Autodesk Inventor part; units mm, degrees
ref_plane "YZ Plane" through (0, 0, 0) normal (1, 0, 0) x (0, 1, 0)
ref_plane "XZ Plane" through (0, 0, 0) normal (0, 1, 0) x (-1, 0, 0)
ref_plane "XY Plane" through (0, 0, 0) normal (0, 0, 1) x (1, 0, 0)
sketch "skt_base" plane through (0, 0, 0) normal (0, 0, 1) x (1, 0, 0)
  line L0 (-30, -8.25) -> (30, -8.25)
  line L1 (30, -8.25) -> (30, 8.25)
  line L2 (30, 8.25) -> (-30, 8.25)
  line L3 (-30, 8.25) -> (-30, -8.25)
  line L4 (-30, -8.25) -> (30, 8.25) construction
  line L5 (30, -8.25) -> (-30, 8.25) construction
  line L6 (-30, 0) -> (30, 0) construction
  line L7 (0, -8.25) -> (0, 8.25) construction
  line L8 (14.5, 0) -> (23.5, 0) construction
  line L9 (16.75, -2.25) -> (21.25, -2.25)
  line L10 (21.25, 2.25) -> (16.75, 2.25)
  arc A0 (16.75, 2.25) -> (16.75, -2.25) centre (16.75, 0) ccw
  arc A1 (21.25, -2.25) -> (21.25, 2.25) centre (21.25, 0) ccw
  line L11 (12.5, 0) -> (25.5, 0) construction
  line L12 (16.75, -4.25) -> (21.25, -4.25)
  line L13 (21.25, 4.25) -> (16.75, 4.25)
  arc A2 (16.75, 4.25) -> (16.75, -4.25) centre (16.75, 0) ccw
  arc A3 (21.25, -4.25) -> (21.25, 4.25) centre (21.25, 0) ccw
  line L14 (-16.75, -2.25) -> (-21.25, -2.25)
  line L15 (-21.25, 2.25) -> (-16.75, 2.25)
  arc A4 (-16.75, -2.25) -> (-16.75, 2.25) centre (-16.75, 0) ccw
  arc A5 (-21.25, 2.25) -> (-21.25, -2.25) centre (-21.25, 0) ccw
  line L16 (-16.75, -4.25) -> (-21.25, -4.25)
  line L17 (-21.25, 4.25) -> (-16.75, 4.25)
  arc A6 (-16.75, -4.25) -> (-16.75, 4.25) centre (-16.75, 0) ccw
  arc A7 (-21.25, 4.25) -> (-21.25, -4.25) centre (-21.25, 0) ccw
  circle A8 centre (0, 0) radius 3.75
  circle A9 centre (0, 0) radius 6
  circle A10 centre (0, 0) radius 8
  point P0 (0, 0)
  point P1 (19, 0)
  point P2 (19, 0)
  point P3 (0, 0)
  dimension "d13" = 60
  dimension "d14" = 16.5
  dimension "d29" = 6.5
  dimension "d30" = 4.5
  dimension "d31" = 9
  dimension "d32" = 2
  dimension "d33" = 2
  dimension "d47" = 16
  dimension "d48" = 12
  dimension "d49" = 7.5
extrude "base" add sketch "skt_base" along normal blind 3.5 contours L3 L2 L1 L0
extrude "screw_head" add sketch "skt_base" along normal blind 1.75 contours A2 L13 A3 L12 | L16 A7 L17 A6
extrude "handle_support" add sketch "skt_base" along normal blind 7 contours A10
extrude "handle_guide" add sketch "skt_base" along normal blind 5.5 contours A9
extrude "handle_screw_head" cut sketch "skt_base" along normal blind 3.7 contours A9
fillet "side_fillets" radius 4 4 edges at (-30, -8.25, 1.75) (30, -8.25, 1.75) (30, 8.25, 1.75) (-30, 8.25, 1.75)
equation "\"d13\" = base_l"
equation "\"d14\" = base_w"
equation "\"d29\" = base_screw_b"
equation "\"d30\" = base_screw_w"
equation "\"d31\" = base_screw_l"
equation "\"d32\" = base_screw_p"
equation "\"d33\" = base_screw_p"
equation "\"d47\" = handle_screw_e"
equation "\"d48\" = handle_screw_p"
equation "\"d49\" = handle_screw_d"
equation "\"d15\" = base_t"
equation "\"d34\" = base_screw_t"
equation "\"d50\" = handle_screw_h"
equation "\"d52\" = handle_screw_h - handle_screw_b"
equation "\"d54\" = handle_screw_h - 2.2 * handle_screw_b"
equation "\"wall_inner_diam\" = 2"
equation "\"wall_outer_diam\" = 1"
equation "\"wall_height\" = 8"
equation "\"leg_diam\" = 3"
equation "\"leg_height\" = 4"
equation "\"wall_widh\" = 8"
equation "\"base_screw_w\" = 4.5"
equation "\"base_t\" = 3.5"
equation "\"base_w\" = 16.5"
equation "\"base_l\" = 60"
equation "\"base_screw_p\" = 2"
equation "\"base_screw_l\" = 9"
equation "\"base_screw_t\" = 1.75"
equation "\"base_screw_b\" = 6.5"
equation "\"handle_screw_p\" = 12"
equation "\"handle_screw_d\" = 7.5"
equation "\"handle_screw_e\" = 16"
equation "\"handle_screw_b\" = 1.5"
equation "\"handle_screw_h\" = 7"
equation "\"d44\" = 7.5"
equation "\"d45\" = 16"
equation "\"d46\" = 12"
properties part number "coffee"
Could you check a few things on this model? Use its own coordinates, in mm. A direction names the side the tool comes from. Coordinates: 2 decimals unless noted, no trailing zeros. Write each loop counter-clockwise with the first axis right and the second up, starting at its lowest first coordinate (ties: lowest second). Pieces come first, ordered by that corner, then holes. Notation, with made-up numbers: (18.25, 74.5) - (57.25, 74.5) arc R22 ccw to (57.25, 93.5) - close; hole circle Ø9 at (-22, 23.25). An arc over 180 degrees is marked (long way). Put each result on its own line as item: value. Start each with the question number.
Q1. I want a section at C-C on x = -11.5. Write out the boundary of the cut face in (y, z).
Q2. I want a section at B-B on x = 2.5. Write out the boundary of the cut face in (y, z).
Q3. Thinking about a two-plate mould opening in Y: for faces 1 (the cylindrical face through (23.5, 0, 0.9)), 2 (the cylindrical face through (28.859, 7.047, 1.774)), 3 (the flat face through (-2, 6, 7)), which applies, pulls with the +Y half, pulls with the -Y half, needs draft (parallel to the pull), parting line crosses it, or undercut?
Q4. I want a section at A-A on z = 1. Write out the boundary of the cut face in (x, y).
Q5. Please list where these lines run through material, in increasing order: L1, parallel to X at y = 1.75, z = 3; L2, parallel to Y at x = 0, z = 2.8; L3, parallel to Z at x = 18.5, y = 6.75.
Q6. I'm going to push flat-ended pins straight in: P1, Ø3.5, axis at x = -0.5, y = -1.5, coming from the +Z side; P2, Ø1.5, axis at y = 5.5, z = 3.5, coming from the -X side; P3, Ø9.5, axis at x = -18, y = 1.5, coming from the +Z side; P4, Ø6, axis at x = -1.5, y = -1, coming from the -Z side. Where does each tip first touch, or does it pass through?
Q7. Which directions (+Z, -Z, +X, -X, +Y, -Y) give clear straight access to the entire face, cutting with the end or side of a thin tool? Please do faces 4 (the cylindrical face through (-6, 0, 2)), 5 (the flat face through (-30, 0, 2)), 6 (the cylindrical face through (-28.797, 7.109, 1.774)), 7 (the flat face through (19, -2.25, 1)), 8 (the flat face through (-19, -3, 1.75)).
Checks:
1. outline: (-8.25, 0) - (8.25, 0) - (8.25, 3.5) - (-8.25, 3.5) - close
2. outline: (-8.25, 0) - (-5.45, 0) - (-5.45, 3.7) - (-2.8, 3.7) - (-2.8, 5.5) - (-5.45, 5.5) - (-5.45, 7) - (-7.6, 7) - (-7.6, 3.5) - (-8.25, 3.5) - close; (2.8, 3.7) - (5.45, 3.7) - (5.45, 0) - (8.25, 0) - (8.25, 3.5) - (7.6, 3.5) - (7.6, 7) - (5.45, 7) - (5.45, 5.5) - (2.8, 5.5) - close
3. face 1: undercut
3. face 2: pulls with the +Y half
3. face 3: needs draft
4. outline: (-30, -4.25) arc R4 ccw to (-26, -8.25) - (26, -8.25) arc R4 ccw to (30, -4.25) - (30, 4.25) arc R4 ccw to (26, 8.25) - (-26, 8.25) arc R4 ccw to (-30, 4.25) - close; hole (-21.25, -2.25) - (-16.75, -2.25) arc R2.25 ccw to (-16.75, 2.25) - (-21.25, 2.25) arc R2.25 ccw to start; hole circle Ø12 at (0, 0); hole (16.75, -2.25) - (21.25, -2.25) arc R2.25 ccw to (21.25, 2.25) - (16.75, 2.25) arc R2.25 ccw to start
5. L1: -30 to -25.12, -12.88 to -5.74, 5.74 to 12.88, 25.12 to 30
5. L2: -8.25 to -6, 6 to 8.25
5. L3: 0 to 3.5
6. P1: through
6. P2: x = -29.97
6. P3: z = 3.5
6. P4: z = 3.7
7. face 4: -Z
7. face 5: +Z, -Z, -X, +Y, -Y
7. face 6: +Z, -Z, -X, +Y
7. face 7: +Z, -Z
7. face 8: +Z
